```python
from build123d import *

# Parameters (mm, degrees)
BOSS_EXTRUDE1_DEPTH          = 12.7
CUT_EXTRUDE1_DEPTH           = 338.387447899
HOLE1_D                      = 30
HOLE2_D                      = 47
F_39_0_0995_DIAMETER_HOLE1_D = 2.5273
F_4_CLEARANCE_HOLE1_D        = 3.3
F_2_CLEARANCE_HOLE1_D        = 2.499999999
F_4_CLEARANCE_HOLE2_D        = 3.3
F_4_CLEARANCE_HOLE2_DEPTH    = 10
SKETCH_1_W                   = 10
SKETCH_1_H                   = 80
CUT_EXTRUDE_1_DEPTH          = 338.387447899
FILLET_1_R                   = 5


with BuildPart() as part:
    # Sketch1 → Boss-Extrude1 (new body)
    with BuildSketch(Plane.XY.offset(12.7)):
        with BuildLine():
            Line((-30, 305), (-30, 23.323807579))
            ThreePointArc((-30, 23.323807579), (0, -38), (30, 23.323807579))
            Line((30, 23.323807579), (30, 305))
            ThreePointArc((30, 305), (0, 335), (-30, 305))
        make_face()
    extrude(amount=-BOSS_EXTRUDE1_DEPTH)

    # Sketch2 → Cut-Extrude1 (cut, through all)
    with BuildSketch(Plane(origin=(0, 0, 0), x_dir=(-1, 0, 0), z_dir=(0, 0, -1))):
        with BuildLine():
            Line((18.5, 69.02247107), (18.5, 84.02247107))
            ThreePointArc((18.5, 84.02247107), (0, 102.52247107), (-18.5, 84.02247107))
            Line((-18.5, 84.02247107), (-18.5, 69.02247107))
            ThreePointArc((-18.5, 69.02247107), (0, 50.52247107), (18.5, 69.02247107))
        make_face()
    extrude(amount=-CUT_EXTRUDE1_DEPTH, mode=Mode.SUBTRACT)

    # Hole1 (through all)
    with Locations(Plane.XY.offset(12.7)):
        with Locations((0, 0)):
            Hole(HOLE1_D / 2)

    # Hole2 (through all)
    with Locations(Plane.XY.offset(12.7)):
        with Locations((0, 305)):
            Hole(HOLE2_D / 2)

    # #39 (0.0995) Diameter Hole1 (through all)
    with Locations(Plane.XY.offset(12.7)):
        with Locations((-26.75, 74.022471071), (-26.75, 129.511235535), (-26.75, 186.111235535), (-26.750000001, 192.911235535), (-26.750000001, 249.511235535), (-26.750000001, 305), (-3.300000001, 331.545668196), (3.299999999, 331.545668196), (26.749999999, 305), (26.749999999, 249.511235535), (26.749999999, 192.911235535), (26.75, 186.111235535), (26.75, 129.511235535), (26.75, 74.022471071), (3.4, 47.489425637), (-3.3, 47.476802874), (-23.166179551, 318.375), (-23.166179551, 291.625), (0, 278.25), (23.166179551, 291.625), (23.166179551, 318.375), (0, 331.75)):
            Hole(F_39_0_0995_DIAMETER_HOLE1_D / 2)

    # #4 Clearance Hole1 (through all)
    with Locations(Plane(origin=(0, 0, 0), x_dir=(-1, 0, 0), z_dir=(0, 0, -1))):
        with Locations((-25.5016, 64.272471071), (-25.5016, 88.772471071), (14.424978336, 14.424978336), (20.4, 0), (14.424978336, -14.424978336), (0, -20.4), (-14.424978336, -14.424978336), (-20.4, 0), (-14.424978336, 14.424978336), (0, 20.4), (25.5016, 64.272471071), (25.5016, 88.772471071)):
            Hole(F_4_CLEARANCE_HOLE1_D / 2)

    # #2 Clearance Hole1 (through all)
    with Locations(Plane(origin=(0, 0, 0), x_dir=(-1, 0, 0), z_dir=(0, 0, -1))):
        with Locations((-1.619921459, 231.265288591), (-21.578861519, 245.43367635)):
            Hole(F_2_CLEARANCE_HOLE1_D / 2)

    # #4 Clearance Hole2
    with Locations(Plane(origin=(30, 0, 0), x_dir=(0, 0, -1), z_dir=(1, 0, 0))):
        with Locations((-6.35, 285.723807579), (-6.35, 133.323807579)):
            Hole(F_4_CLEARANCE_HOLE2_D / 2, depth=F_4_CLEARANCE_HOLE2_DEPTH)

    # 草图1 → 切除-拉伸1 (cut, through all)
    with BuildSketch(Plane(origin=(0, 0, 0), x_dir=(-1, 0, 0), z_dir=(0, 0, -1))):
        with Locations((0, 166.265288591)):
            Rectangle(SKETCH_1_W, SKETCH_1_H)
    extrude(amount=-CUT_EXTRUDE_1_DEPTH, mode=Mode.SUBTRACT)

    # 圆角1
    fillet_1_edges = [part.edges().sort_by_distance(p)[0] for p in [
        (-5, 126.265288591, 6.35),
        (5, 126.265288591, 6.35),
        (-5, 206.265288591, 6.35),
        (5, 206.265288591, 6.35),
    ]]
    fillet(fillet_1_edges, radius=FILLET_1_R - 0.0001)  # a hair under: the kernel refuses the full size


solid = part.part
```
Geometry check sheet. Reference: the model listing, model coordinates, mm. A direction names the side the tool comes from. Round coordinates to 2 decimals unless told otherwise and drop trailing zeros. Order: outer loops, then holes, each group sorted by start corner. A loop starts at its lowest first (then second) coordinate and runs counter-clockwise, first axis right, second up. Notation, with made-up numbers: (-12.75, 19.25) -> (14.25, 19.25) arc R26 cw to (14.25, 37.25) -> close; hole circle Ø9 at (2, 87). An arc over 180 degrees is marked (long way). Return JSON: item names as keys, results as strings. Group by question number.
Q1. Gauge pin test, flat ends, axial feed: pin 1 (3 mm diameter, centred on y = 133.32, z = 6.35, fed in from +X); pin 2 (2 mm diameter, centred on y = 239, z = 8.5, fed in from -X); pin 3 (4 mm diameter, centred on y = 96.5, z = 9, fed in from +X); pin 4 (2 mm diameter, centred on x = 1.62, y = 231.27, fed in from -Z). Record the tip position at first contact, or that the pin passes through.
Q2. Material ranges on probe 1 along X at (y, z) = (297, 2.25); probe 2 along Y at (x, z) = (-12.5, 6.5); probe 3 along X at (y, z) = (138, 6), recorded low to high. Write a range as from..to.
Q3. Tool access check on faces 1 (the flat face through (-18.5, 76, 6)), 2 (the flat face through (8, 151, 0)), 3 (the flat face through (30, 162, 6)), 4 (the flat face through (-30, 166, 6)). Record the directions out of +Z, -Z, +X, -X, +Y, -Y that give a thin tool (end or side, any length) a straight path to the whole face; none if there is none.
Q4. Section check A-A, the plane y = 157.5. Record the boundary of the cut face in (x, z).
Q5. Release check for a two-part mould opening along Y. For faces 5 (the cylindrical face through (3.06, 328.3, 6.26)), 6 (the flat face through (8, 151, 12.7)), 7 (the cylindrical face through (0.66, 334.993, 6.439)) record: released by +Y, released by -Y, zero draft, split by the parting line, or undercut.
Q6. Section check B-B, the plane x = -8.5. Record the boundary of the cut face in (y, z), plus the area to 3 significant figures.
Q7. Section check C-C, the plane y = 7. Record the boundary of the cut face in (x, z), plus the area to 3 significant figures.
Numbers:
{
 "1": {"pin 1": "x = 20", "pin 2": "x = -30", "pin 3": "x = 30", "pin 4": "through"},
 "2": {"probe 1": "-30..-22.1, 22.1..30", "probe 2": "-35.89..-8.29, 8.29..55.38, 97.66..285.1, 324.9..332.27", "probe 3": "-30..-5, 5..30"},
 "3": {"face 1": "+Z, -Z", "face 2": "-Z, +X, -X, +Y, -Y", "face 3": "+Z, -Z, +X, +Y", "face 4": "+Z, -Z, -X, +Y"},
 "4": {"outline": "(-30, 0) -> (-5, 0) -> (-5, 12.7) -> (-30, 12.7) -> close; (5, 0) -> (30, 0) -> (30, 12.7) -> (5, 12.7) -> close"},
 "5": {"face 5": "undercut", "face 6": "zero draft", "face 7": "released by +Y"},
 "6": {"outline": "(-37.04, 0) -> (-12.36, 0) -> (-12.36, 12.7) -> (-37.04, 12.7) -> close; (12.36, 0) -> (52.59, 0) -> (52.59, 12.7) -> (12.36, 12.7) -> close; (100.45, 0) -> (283.09, 0) -> (283.09, 12.7) -> (100.45, 12.7) -> close; (326.91, 0) -> (333.77, 0) -> (333.77, 12.7) -> (326.91, 12.7) -> close", "area": "3,230 mm^2"},
 "7": {"outline": "(-37.35, 0) -> (-13.27, 0) -> (-13.27, 12.7) -> (-37.35, 12.7) -> close; (13.27, 0) -> (37.35, 0) -> (37.35, 12.7) -> (13.27, 12.7) -> close", "area": "612 mm^2"}
}
